from build123d import *

# Parameters (mm, degrees)
F0_W          = 226
F0_H          = 15
F1_DEPTH      = 10
F2_W          = 66
F2_H          = 6
F3_DEPTH      = 7
F4_W          = 85
F4_H          = 49.5
F5_DEPTH      = 3
F5_DEPTH_BACK = 2
F6_W          = 69
F6_H          = 18
F7_DEPTH      = 7
F8_W          = 66
F8_H          = 3
F9_DEPTH      = 25
F10_W         = 85
F10_H         = 1
F11_DEPTH     = 3
F12_W         = 85
F12_H         = 0.5
F13_DEPTH     = 3
F14_R         = 1.5
F15_DEPTH     = 3


with BuildPart() as f1:
    # F0 (on Front) → F1 (new body)
    with BuildSketch(Plane.XZ):
        Rectangle(F0_W, F0_H)
    extrude(amount=F1_DEPTH)

    # F2 (on face) → F3 (join)
    with BuildSketch(Plane.XZ.offset(10)):
        with Locations((0, -4.5)):
            Rectangle(F2_W, F2_H)
    extrude(amount=F3_DEPTH)

    # F4 (on face) → F5 (join, two sides)
    with BuildSketch(Plane(origin=(0, 0, 0), x_dir=(-1, 0, 0), z_dir=(0, 1, 0))) as f5_sk:
        with Locations((0, -24.75)):
            Rectangle(F4_W, F4_H)
    extrude(amount=F5_DEPTH)
    extrude(f5_sk.sketch, amount=-F5_DEPTH_BACK)

    # F6 (on face) → F7 (cut)
    with BuildSketch(Plane(origin=(0, 0, 0), x_dir=(-1, 0, 0), z_dir=(0, 1, 0))):
        with Locations((0, 7.5)):
            Rectangle(F6_W, F6_H)
    extrude(amount=-F7_DEPTH, mode=Mode.SUBTRACT)

    # F8 (on face) → F9 (cut)
    with BuildSketch(Plane(origin=(0, -7, 0), x_dir=(-1, 0, 0), z_dir=(0, 1, 0))):
        with Locations((0, 3)):
            Rectangle(F8_W, F8_H)
    extrude(amount=-F9_DEPTH, mode=Mode.SUBTRACT)

    # F10 (on face) → F11 (cut)
    with BuildSketch(Plane(origin=(0, 3, 0), x_dir=(-1, 0, 0), z_dir=(0, 1, 0))):
        with Locations((0, -0.5)):
            Rectangle(F10_W, F10_H)
    extrude(amount=-F11_DEPTH, mode=Mode.SUBTRACT)

    # F12 (on face) → F13 (cut)
    with BuildSketch(Plane(origin=(0, 3, 0), x_dir=(-1, 0, 0), z_dir=(0, 1, 0))):
        with Locations((0, -1.25)):
            Rectangle(F12_W, F12_H)
    extrude(amount=-F13_DEPTH, mode=Mode.SUBTRACT)

    # F14 (on face) → F15 (join)
    with BuildSketch(Plane(origin=(0, 3, 0), x_dir=(-1, 0, 0), z_dir=(0, 1, 0))):
        with Locations((6, -6)):
            Circle(F14_R)
        with Locations((6, -12)):
            Circle(F14_R)
    extrude(amount=F15_DEPTH)


solid = f1.part
Source: CAD feature listing. Evaluate the final solid. Frame: model axes, mm. A direction names the side the tool comes from. Give positions to 0.01 mm unless a question says otherwise; leave off trailing zeros. Write each loop counter-clockwise with the first axis right and the second up, starting at its lowest first coordinate (ties: lowest second). Pieces come first, ordered by that corner, then holes. Notation, with made-up numbers: M 17,55.5 L 54,55.5 A8 cw 54,70.5 Z; hole C -4.75,34.5 d2. An arc over 180 degrees is marked long. Return JSON: item names as keys, results as strings. Group by question number.
1) Cut plane A-A, the plane x = -2.5. Output: boundary loops of the cut face in (y, z).
2) Set-up query: faces 4 (the face through (-33, -13, -5)), 5 (the face through (0, -13, -1.5)), 6 (the face through (1, -2, -28)), 7 (the face through (-34.5, -3, 3)), 8 (the face through (33, -13, -5)). Return all of +Z, -Z, +X, -X, +Y, -Y with unobstructed straight access to the full face (end or side cutting, diameter ignored); none if empty.
3) Draft query along X for faces 1 (the face through (-1.6, -7.2, 7.5)), 2 (the face through (113, -5, 0)), 3 (the face through (1, -2, -1.5)). Return one class per face: released by +X, released by -X, zero draft, split by the parting line, or undercut.
4) First-contact query: pin 1 Ø5.5 at (x, y) = (-7.5, -15) entering from +Z; pin 2 Ø6 at (y, z) = (-2.5, -26) entering from +X; pin 3 Ø1.5 at (x, y) = (-24, -9.5) entering from -Z. Flat tips, straight axial feed; report the tip coordinate or a pass-through.
5) Cut plane D-D, the plane y = -13. Output: boundary loops of the cut face in (x, z).
6) Ray query, L1, parallel to X at y = -6.25, z = 0; L2, parallel to Z at x = -23, y = -9.75; L3, parallel to Z at x = -11, y = -15.25. Return the intervals inside material, ascending.
7) Cut plane C-C, the plane z = -43.5. Output: boundary loops of the cut face in (x, y), then the cut area to 3 significant figures.
8) Cut plane B-B, the plane x = 39.5. Output: boundary loops of the cut face in (y, z), then the cut area to 3 significant figures.
Data:
{
 "1": {"outline": "M -17,-7.5 L -2,-7.5 L -2,-49.5 L 3,-49.5 L 3,-1.5 L -7,-1.5 L -7,1.5 L -10,1.5 L -10,-1.5 L -17,-1.5 Z; M -10,4.5 L -7,4.5 L -7,7.5 L -10,7.5 Z"},
 "2": {"face 4": "+Z, -Z, -X, -Y", "face 5": "+Z, +X, -X, -Y", "face 6": "-Z, +X, -X, -Y", "face 7": "+Z, +Y", "face 8": "+Z, -Z, +X, -Y"},
 "3": {"face 1": "zero draft", "face 2": "released by +X", "face 3": "undercut"},
 "4": {"pin 1": "stops at z = -1.5", "pin 2": "stops at x = 42.5", "pin 3": "stops at z = -7.5"},
 "5": {"outline": "M -33,-7.5 L 33,-7.5 L 33,-1.5 L -33,-1.5 Z"},
 "6": {"L1": "x = -113 to -34.5, 34.5 to 113", "L2": "z = -7.5 to 1.5, 4.5 to 7.5", "L3": "z = -7.5 to -1.5"},
 "7": {"outline": "M -42.5,-2 L 42.5,-2 L 42.5,3 L -42.5,3 Z", "area": "425 mm²"},
 "8": {"outline": "M -10,-7.5 L -2,-7.5 L -2,-49.5 L 3,-49.5 L 3,-1.5 L 0,-1.5 L 0,7.5 L -10,7.5 Z", "area": "378 mm²"}
}
